Could you check a few things on this drawing? It's one solid part, dimensions in mm from its lowest x, y, z. Give positions to 0.01 mm unless a question says otherwise; leave off trailing zeros. Write each loop counter-clockwise with the first axis right and the second up, starting at its lowest first coordinate (ties: lowest second). Pieces come first, ordered by that corner, then holes. Notation, with made-up numbers: M 70.25,-19.75 L 115.25,-19.75 A20 ccw 115.25,18.25 Z; hole C 40,21.25 d10. An arc over 180 degrees is marked long. Use CSV: the item, a comma, the result in double quotes. Start each with the question number.
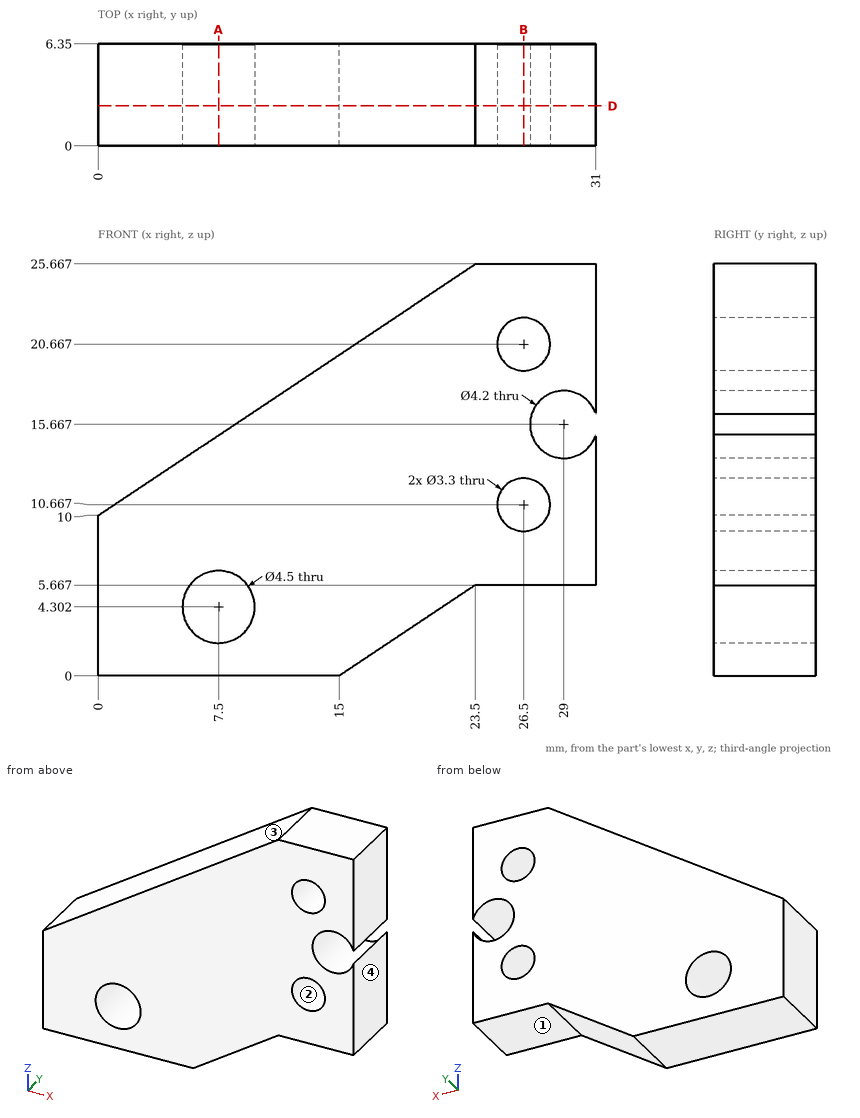
(1) Thinking about a two-plate mould opening in Z: for the marked faces 1, 2, 3 and 4, which applies, released by +Z, released by -Z, zero draft, split by the parting line, or undercut?
(2) Will these pins go through, and if not, where does the flat tip stop? pin 1 Ø3 at (y, z) = (5, 19.5) entering from -X; pin 2 Ø3 at (x, y) = (26.5, 4) entering from -Z; pin 3 Ø3 at (x, y) = (22.5, 2) entering from -Z.
(3) I want a section at A-A (x = 7.5). Write out the boundary of the cut face in (y, z).
(4) I want a section at B-B (x = 26.5). Write out the boundary of the cut face in (y, z).
(5) I want a section at D-D (y = 2.5). Write out the boundary of the cut face in (x, z).
(6) Please list where these lines run through material, in increasing order: L1, parallel to Z at x = 26.5, y = 2.5; L2, parallel to Z at x = 7.5, y = 1.75; L3, parallel to Z at x = 7, y = 3.5 (1 decimal). Write a range as [from, to].
Geometry results:
1,face 1,"released by -Z"
1,face 2,"undercut"
1,face 3,"released by +Z"
1,face 4,"zero draft"
2,pin 1,"stops at x = 12"
2,pin 2,"stops at z = 5.67"
2,pin 3,"stops at z = 4"
3,outline,"M 0,0 L 6.35,0 L 6.35,2.05 L 0,2.05 Z; M 0,6.55 L 6.35,6.55 L 6.35,15 L 0,15 Z"
4,outline,"M 0,5.67 L 6.35,5.67 L 6.35,9.02 L 0,9.02 Z; M 0,12.32 L 6.35,12.32 L 6.35,19.02 L 0,19.02 Z; M 0,22.32 L 6.35,22.32 L 6.35,25.67 L 0,25.67 Z"
5,outline,"M 0,0 L 15,0 L 23.5,5.67 L 31,5.67 L 31,15.03 A2.1 cw long 31,16.31 L 31,25.67 L 23.5,25.67 L 0,10 Z; hole C 7.5,4.3 d4.5; hole C 26.5,10.67 d3.3; hole C 26.5,20.67 d3.3"
6,L1,"z = [5.67, 9.02], [12.32, 19.02], [22.32, 25.67]"
6,L2,"z = [0, 2.05], [6.55, 15]"
6,L3,"z = [0, 2.1], [6.5, 14.7]"
